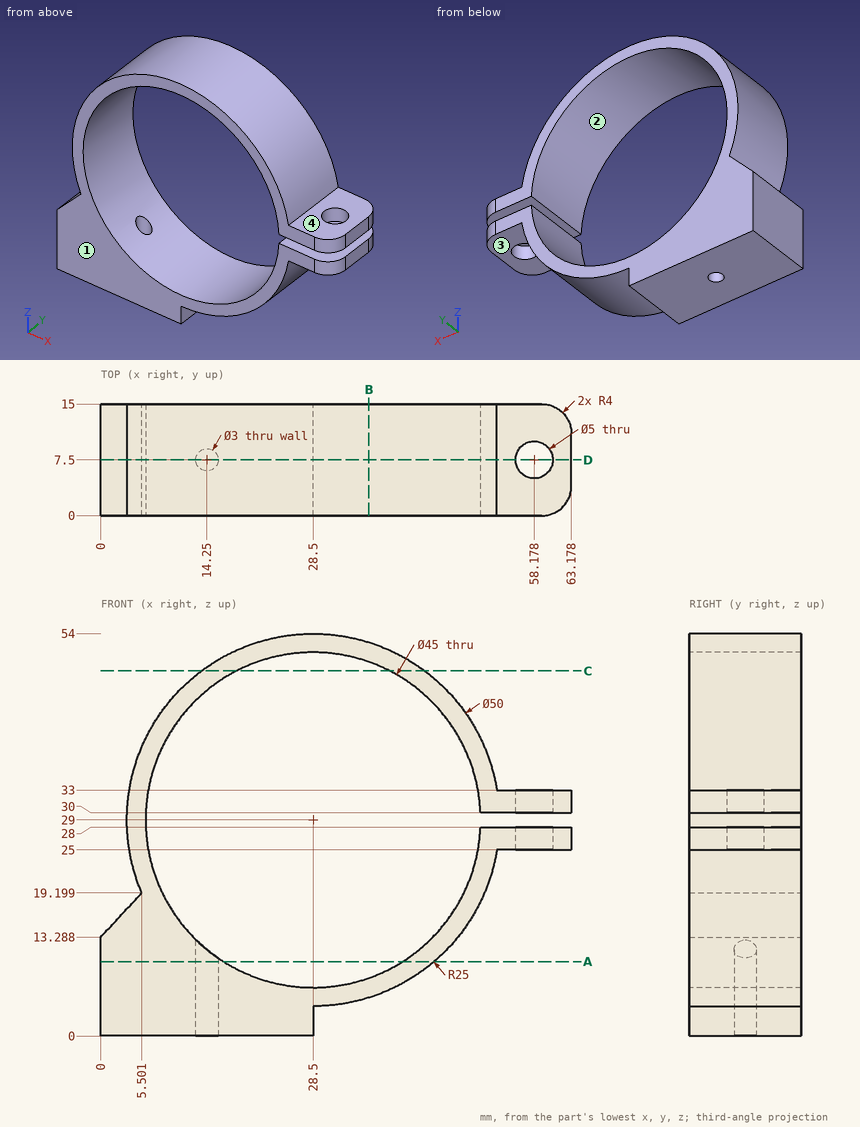
The drawing under review shows one solid part. Ordinate dimensions are in mm from its lowest x, y, z. Coordinates: 2 decimals unless noted, no trailing zeros. Order: outer loops, then holes, each group sorted by start corner. A loop starts at its lowest first (then second) coordinate and runs counter-clockwise, first axis right, second up. Notation, with made-up numbers: (77, 55.25) -> (116, 55.25) arc R15 ccw to (116, 71.25) -> close; hole circle Ø1 at (66.25, 32). An arc over 180 degrees is marked (long way). One line per item, written item: value.
1) Draft analysis for pull direction Z (two halves, no side actions). For the marked faces 1, 2, 3 and 4, state which applies: +Z half, -Z half, draft (parallel to the pull), parting line (faces both ways), or undercut.
Output values:
face 1: draft
face 2: undercut
face 3: -Z half
face 4: +Z half
2) We need section A-A, the plane z = 10. Give the boundary of the cut face in (x, y).
Output values:
outline: (0, 0) -> (16.45, 0) -> (16.45, 15) -> (0, 15) -> close; (40.55, 0) -> (44.75, 0) -> (44.75, 15) -> (40.55, 15) -> close; hole circle Ø3 at (14.25, 7.5)
3) Clearance check with flat-ended pins moving along their axes: P1, Ø2, axis at x = 56, y = 9.5, coming from the -Z side; P2, Ø3, axis at y = 8, z = 1.5, coming from the +X side; P3, Ø3, axis at x = 51, y = 9.5, coming from the +Z side (1 decimal). State where each tip first meets the part, or that it passes through.
Output values:
P1: stops at z = 25
P2: stops at x = 28.5
P3: stops at z = 42.6
4) We need section B-B, the plane x = 36. Give the boundary of the cut face in (y, z).
Output values:
outline: (0, 5.15) -> (15, 5.15) -> (15, 7.79) -> (0, 7.79) -> close; (0, 50.21) -> (15, 50.21) -> (15, 52.85) -> (0, 52.85) -> close
5) We need section D-D, the plane y = 7.5. Give the boundary of the cut face in (x, z).
Output values:
outline: (0, 0) -> (12.75, 0) -> (12.75, 12.93) arc R22.5 cw (long way) to (50.98, 30) -> (55.68, 30) -> (55.68, 33) -> (53.18, 33) arc R25 ccw (long way) to (5.5, 19.2) -> (0, 13.29) -> close; (15.75, 0) -> (28.5, 0) -> (28.5, 4) arc R25 ccw to (53.18, 25) -> (55.68, 25) -> (55.68, 28) -> (50.98, 28) arc R22.5 cw to (15.75, 10.46) -> close; (60.68, 25) -> (63.18, 25) -> (63.18, 28) -> (60.68, 28) -> close; (60.68, 30) -> (63.18, 30) -> (63.18, 33) -> (60.68, 33) -> close
6) To check wall thickness, follow probe 1 along Z at (x, y) = (54, 1.5); probe 2 along Y at (x, z) = (14.25, 4.75); probe 3 along Y at (x, z) = (60, 31.5) (1 decimal). State the ranges of each line that lie inside material, in increasing order. Write a range as [from, to].
Output values:
probe 1: z = [25, 28], [30, 33]
probe 2: y = [0, 6], [9, 15]
probe 3: y = [0.1, 5.8], [9.2, 14.9]
7) We need section C-C, the plane z = 49. Give the boundary of the cut face in (x, y).
Output values:
outline: (13.5, 0) -> (18.19, 0) -> (18.19, 15) -> (13.5, 15) -> close; (38.81, 0) -> (43.5, 0) -> (43.5, 15) -> (38.81, 15) -> close
